Part model, mm, in its own coordinate system. Face numbers are marked on the shaded views. A direction names the side the tool comes from. Give positions to 0.01 mm unless a question says otherwise; leave off trailing zeros. Loops run counter-clockwise (first coordinate to the right, second up) from the corner with the lowest first, then second, coordinate; pieces in that order, holes last. Notation, with made-up numbers: (72.25, 29.5) -> (123.25, 29.5) arc R15 cw to (123.25, 44.5) -> close; hole circle Ø1 at (-33, 34.5). An arc over 180 degrees is marked (long way). One line per question, with ' | ' between items.
```python
from build123d import *

# Parameters (mm, degrees)
SKETCH_R        = 4.2
PAD_DEPTH       = 8
SKETCH002_W     = 6
SKETCH002_H     = 2.5
POCKET001_DEPTH = 8.001
SKETCH003_R     = 2.65
POCKET_DEPTH    = 57.001
FILLET_R        = 3
CHAMFER_SIZE    = 0.5
FILLET001_R     = 1


with BuildPart() as part:
    # Sketch → Pad (new body)
    with BuildSketch(Plane.XY):
        with BuildLine():
            Line((-8.746857, 7), (-27, 7))
            Line((-27, 7), (-27, 0))
            Line((-27, 0), (27, 0))
            Line((27, 0), (27, 7))
            Line((8.746857, 7), (27, 7))
            Line((5.80237, 12.1), (8.746857, 7))
            ThreePointArc((5.80237, 12.1), (0, 15.45), (-5.80237, 12.1))
            Line((-8.746857, 7), (-5.80237, 12.1))
        make_face()
        with Locations((0, 8.75)):
            Circle(SKETCH_R, mode=Mode.SUBTRACT)
    extrude(amount=PAD_DEPTH)

    # Sketch002 → Pocket001 (cut, through all)
    with BuildSketch(Plane(origin=(0, 0, 0), x_dir=(1, 0, 0), z_dir=(0, 0, -1))):
        with Locations((0, -1.25)):
            Rectangle(SKETCH002_W, SKETCH002_H)
    extrude(amount=-POCKET001_DEPTH, mode=Mode.SUBTRACT)

    # Sketch003 → Pocket (cut, through all)
    with BuildSketch(Plane(origin=(-30, 0, 0), x_dir=(0, -1, 0), z_dir=(-1, 0, 0))):
        with Locations((0.75, 4)):
            Circle(SKETCH003_R)
    extrude(amount=-POCKET_DEPTH, mode=Mode.SUBTRACT)

    # Fillet
    fillet_edges = [part.edges().sort_by_distance(p)[0] for p in [
        (-8.746857, 7, 4),
        (8.746857, 7, 4),
    ]]
    fillet(fillet_edges, radius=FILLET_R)

    # Chamfer
    chamfer_edges = [part.edges().sort_by_distance(p)[0] for p in [
        (-18.739454, 7, 8),
        (-18.739454, 7, 0),
    ]]
    chamfer(chamfer_edges, length=CHAMFER_SIZE)

    # Fillet001
    fillet001_edges = [part.edges().sort_by_distance(p)[0] for p in [
        (-3, 2.5, 4),
        (3, 2.5, 4),
    ]]
    fillet(fillet001_edges, radius=FILLET001_R)


solid = part.part
```
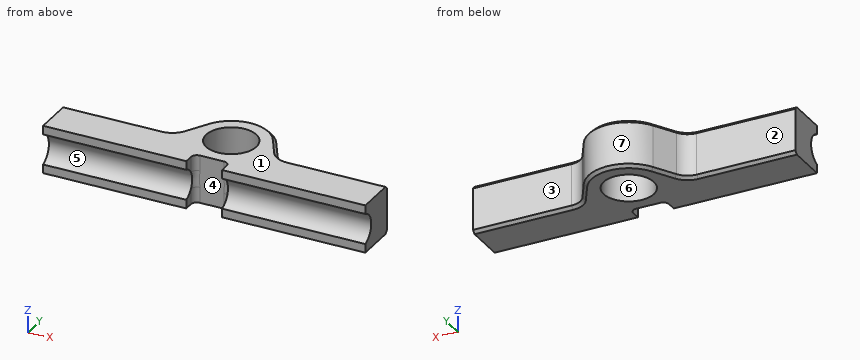
1) Saw through at B-B (y = 5.25). Give the cut face in (x, z).
Found:
outline: (-27, 0) -> (-2.32, 0) -> (-2.32, 8) -> (-27, 8) -> close; (2.32, 0) -> (27, 0) -> (27, 8) -> (2.32, 8) -> close
2) Saw through at A-A (x = 0). Give the cut face in (y, z).
Found:
outline: (2.5, 0) -> (4.55, 0) -> (4.55, 8) -> (2.5, 8) -> close; (12.95, 0) -> (14.95, 0) -> (15.45, 0.5) -> (15.45, 7.5) -> (14.95, 8) -> (12.95, 8) -> close
3) Saw through at D-D (x = 24.5). Give the cut face in (y, z).
Found:
outline: (0, 0) -> (6.5, 0) -> (7, 0.5) -> (7, 7.5) -> (6.5, 8) -> (0, 8) -> (0, 6.54) arc R2.65 cw to (0, 1.46) -> close
4) Drill centre lines: line 1 (Y direction, x = 0, z = 3.25); line 2 (Y direction, x = -16, z = 3.75); line 3 (X direction, y = 11.5, z = 5). Where is each one in solid material? Low to high.
Found:
line 1: 2.5 to 4.55, 12.95 to 15.45 | line 2: 1.89 to 7 | line 3: -6.15 to -3.17, 3.17 to 6.15
5) Saw through at C-C (z = 1). Give the cut face in (x, y).
Found:
outline: (-27, 0) -> (-3, 0) -> (-3, 1.5) arc R1 cw to (-2, 2.5) -> (2, 2.5) arc R1 cw to (3, 1.5) -> (3, 0) -> (27, 0) -> (27, 7) -> (10.48, 7) arc R3 cw to (7.88, 8.5) -> (5.8, 12.1) arc R6.7 ccw to (-5.8, 12.1) -> (-7.88, 8.5) arc R3 cw to (-10.48, 7) -> (-27, 7) -> close; hole circle Ø8.4 at (0, 8.75)
6) Tool access for the marked faces 1, 2, 3 and 4: list every direction of +Z, -Z, +X, -X, +Y, -Y with a clear straight run to the whole face (end or side of a thin tool).
Found:
face 1: +Z, +X, -X, +Y, -Y | face 2: +Z, -Z, -X, +Y | face 3: +Z, -Z, +X, +Y | face 4: +Z, -Z, -Y
7) Pin check, flat tips, straight feed: P1, Ø1, axis at y = 11, z = 3.5, coming from the -X side; P2, Ø1.5, axis at x = 11.5, z = 1.5, coming from the +Y side; P3, Ø1.3, axis at x = 0, z = 5, coming from the -Y side. Stop position of each tip, or through.
Found:
P1: x = -6.73 | P2: y = 7 | P3: y = 2.5
8) Pull direction Y, two halves, no side cores. Call the marked faces 5, 6 and 7: pulls with the +Y half, pulls with the -Y half, needs draft (parallel to the pull), parting line crosses it, or undercut.
Found:
face 5: pulls with the -Y half | face 6: undercut | face 7: pulls with the +Y half
